The listing builds one solid part. Answer for the finished solid, in the listing's coordinates (mm). Face numbers are marked on the shaded views. A direction names the side the tool comes from. Coordinates: 2 decimals unless noted, no trailing zeros. Order: outer loops, then holes, each group sorted by start corner. A loop starts at its lowest first (then second) coordinate and runs counter-clockwise, first axis right, second up. Notation, with made-up numbers: (22, 7.5) -> (63, 7.5) arc R26 ccw to (63, 31.5) -> close; hole circle Ø6 at (57.25, -18.5). An arc over 180 degrees is marked (long way). Return JSON: item names as keys, results as strings.
Autodesk Fusion 360 part; units mm, degrees
sketch "Sketch1" plane through (0, 0, 0) normal (0, 0, 1) x (1, 0, 0)
  line L0 (10, -10) -> (-10, -10)
  line L1 (-10, -10) -> (-10, 10)
  line L2 (-10, 10) -> (10, 10)
  line L3 (10, 10) -> (10, -10)
  line L4 (10, -10) -> (-10, 10) construction
  line L5 (-10, -10) -> (10, 10) construction
  dimension "d1" = 20
  dimension "d2" = 20
extrude "Extrude1" add sketch "Sketch1" along normal mid plane 20
sketch "Sketch2" plane through (0, 0, 10) normal (0, 0, 1) x (-1, 0, 0)
  line L0 (-10, -10) -> (10, -10)
  line L1 (10, -10) -> (10, 10)
  line L2 (10, 10) -> (-10, 10)
  line L3 (-10, 10) -> (-10, -10)
  circle A0 centre (0, 0) radius 2
  dimension "d5" = 4
extrude "Extrude2" cut sketch "Sketch2" against normal blind 1 contours A0
sketch "Sketch3" plane through (0, -10, 0) normal (0, -1, 0) x (1, 0, 0)
  line L0 (10, -10) -> (10, 10)
  line L1 (10, 10) -> (-10, 10)
  line L2 (-10, 10) -> (-10, -10)
  line L3 (-10, -10) -> (10, -10)
  line L4 (-10, 10) -> (10, -10) construction
  circle A0 centre (0, 0) radius 2
  circle A1 centre (-5, 5) radius 2
  circle A2 centre (5, -5) radius 2
  dimension "d8" = 4
  dimension "d9" = 4
  dimension "d10" = 4
extrude "Extrude3" cut sketch "Sketch3" against normal blind 1 contours A0 | A1 | A2
sketch "Sketch4" plane through (-10, 0, 0) normal (-1, 0, 0) x (0, -1, 0)
  line L0 (10, -10) -> (10, 10)
  line L1 (10, 10) -> (-10, 10)
  line L2 (-10, 10) -> (-10, -10)
  line L3 (-10, -10) -> (10, -10)
  line L4 (-10, 10) -> (10, -10) construction
  line L5 (10, 10) -> (-10, -10) construction
  circle A0 centre (0, 0) radius 2
  circle A1 centre (-5, 5) radius 2
  circle A2 centre (5, 5) radius 2
  circle A3 centre (-5, -5) radius 2
  circle A4 centre (5, -5) radius 2
  dimension "d13" = 4
  dimension "d14" = 4
  dimension "d15" = 4
  dimension "d16" = 4
extrude "Extrude4" cut sketch "Sketch4" against normal blind 1 contours A0 | A1 | A2 | A3 | A4
sketch "Sketch5" plane through (0, 10, 0) normal (0, 1, 0) x (-1, 0, 0)
  line L0 (10, -10) -> (10, 10)
  line L1 (10, 10) -> (-10, 10)
  line L2 (-10, 10) -> (-10, -10)
  line L3 (-10, -10) -> (10, -10)
  line L4 (-10, 10) -> (10, -10) construction
  circle A0 centre (-5, 5) radius 2
  circle A1 centre (5, -5) radius 2
  dimension "d19" = 4
  dimension "d20" = 4
extrude "Extrude5" cut sketch "Sketch5" against normal blind 1 contours A0 | A1
sketch "Sketch6" plane through (10, 0, 0) normal (1, 0, 0) x (0, 1, 0)
  line L0 (10, -10) -> (10, 10)
  line L1 (10, 10) -> (-10, 10)
  line L2 (-10, 10) -> (-10, -10)
  line L3 (-10, -10) -> (10, -10)
  line L4 (-10, 10) -> (10, -10) construction
  line L5 (10, 10) -> (-10, -10) construction
  line L6 (-10, 0) -> (10, 0) construction
  line L7 (0, 10) -> (0, -10) construction
  circle A0 centre (-5, 0) radius 2
  circle A1 centre (-5, 5) radius 2
  circle A2 centre (-5, -5) radius 2
  circle A3 centre (5, 5) radius 2
  circle A4 centre (5, 0) radius 2
  circle A5 centre (5, -5) radius 2
  dimension "d23" = 4
  dimension "d24" = 4
  dimension "d25" = 4
  dimension "d26" = 4
  dimension "d27" = 4
  dimension "d28" = 4
extrude "Extrude6" cut sketch "Sketch6" against normal blind 1 contours A0 | A1 | A2 | A3 | A4 | A5
sketch "Sketch7" plane through (0, 0, -10) normal (0, 0, -1) x (1, 0, 0)
  line L0 (-10, -10) -> (10, -10)
  line L1 (10, -10) -> (10, 10)
  line L2 (10, 10) -> (-10, 10)
  line L3 (-10, 10) -> (-10, -10)
  line L4 (10, 10) -> (-10, -10) construction
  line L5 (10, -10) -> (-10, 10) construction
  circle A0 centre (5, 5) radius 2
  circle A1 centre (-5, -5) radius 2
  circle A2 centre (-5, 5) radius 2
  circle A3 centre (5, -5) radius 2
  dimension "d31" = 4
  dimension "d32" = 4
  dimension "d33" = 4
extrude "Extrude7" cut sketch "Sketch7" against normal blind 1 contours A0 | A1 | A2 | A3
equation "d1 = diceSize"
equation "d2 = diceSize"
equation "d3 = diceSize"
equation "diceSize = 20 mm"
equation "DivotDia = 4 mm"
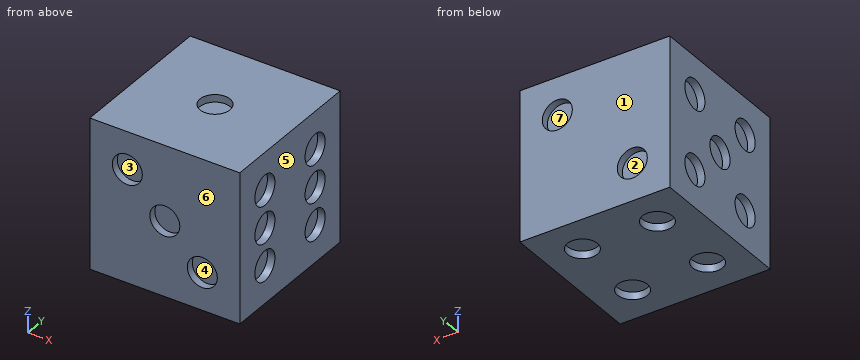
Item 1: The part is cut by section B-B on z = 5. Determine the outline of the cut face in (x, y).
Answer list:
{"outline": "(-10, -10) -> (-7, -10) -> (-7, -9) -> (-3, -9) -> (-3, -10) -> (10, -10) -> (10, -7) -> (9, -7) -> (9, -3) -> (10, -3) -> (10, 3) -> (9, 3) -> (9, 7) -> (10, 7) -> (10, 10) -> (7, 10) -> (7, 9) -> (3, 9) -> (3, 10) -> (-10, 10) -> (-10, 7) -> (-9, 7) -> (-9, 3) -> (-10, 3) -> (-10, -3) -> (-9, -3) -> (-9, -7) -> (-10, -7) -> close"}
Item 2: Flat-ended cylindrical pins translate along their axes: pin 1 (3 mm diameter, centred on x = -5, y = -5, fed in from -Z); pin 2 (3 mm diameter, centred on y = -5, z = -5, fed in from -X); pin 3 (2 mm diameter, centred on x = 4.5, z = 5, fed in from +Y). Find the tip coordinate at first contact, or state that the pin passes through.
Answer list:
{"pin 1": "z = -9", "pin 2": "x = -9", "pin 3": "y = 9"}
Item 3: Find the intervals of material crossed by probe 1 along Z at (x, y) = (9.25, -5); probe 2 along X at (y, z) = (5, -9.8), in increasing order.
Answer list:
{"probe 1": "-10 to -7, -3 to -2, 2 to 3, 7 to 10", "probe 2": "-10 to -7, -3 to 3, 7 to 10"}
Item 4: The part is cut by section C-C on x = -0.75. Determine the outline of the cut face in (y, z).
Answer list:
{"outline": "(-10, -10) -> (10, -10) -> (10, 10) -> (1.85, 10) -> (1.85, 9) -> (-1.85, 9) -> (-1.85, 10) -> (-10, 10) -> (-10, 1.85) -> (-9, 1.85) -> (-9, -1.85) -> (-10, -1.85) -> close"}
Item 5: Determine the mould class of the marked faces 4, 5, 6 and 7 for opening direction X: pulls with the +X half, pulls with the -X half, needs draft (parallel to the pull), parting line crosses it, or undercut.
Answer list:
{"face 4": "undercut", "face 5": "pulls with the +X half", "face 6": "needs draft", "face 7": "undercut"}
Item 6: The part is cut by section D-D on x = 3.5. Determine the outline of the cut face in (y, z).
Answer list:
{"outline": "(-10, -10) -> (-6.32, -10) -> (-6.32, -9) -> (-3.68, -9) -> (-3.68, -10) -> (3.68, -10) -> (3.68, -9) -> (6.32, -9) -> (6.32, -10) -> (10, -10) -> (10, 3.68) -> (9, 3.68) -> (9, 6.32) -> (10, 6.32) -> (10, 10) -> (-10, 10) -> (-10, -3.68) -> (-9, -3.68) -> (-9, -6.32) -> (-10, -6.32) -> close"}
Item 7: Which of the six approach directions +Z, -Z, +X, -X, +Y, -Y give full straight-line access (tool end or side, diameter ignored) to the marked faces 1, 2 and 3?
Answer list:
{"face 1": "+Z, -Z, +X, -X, +Y", "face 2": "+Y", "face 3": "-Y"}
